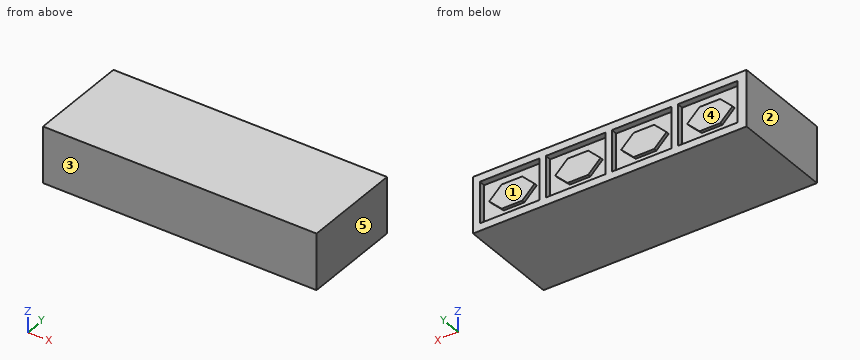
```python
from build123d import *

# Parameters (mm, degrees)
SKETCH2_W           = 132.68
SKETCH2_H           = 48.96
BOSS_EXTRUDE1_DEPTH = 27.2
SKETCH3_W           = 29
SKETCH3_H           = 20
CUT_EXTRUDE1_DEPTH  = 3
SKETCH4_W           = 10
SKETCH4_H           = 11.64
BOSS_EXTRUDE2_DEPTH = 1.5
LPATTERN1_COUNT     = 4
LPATTERN1_PITCH     = 32


with BuildPart() as part:
    # Sketch2 → Boss-Extrude1 (new body)
    with BuildSketch(Plane.XY):
        with Locations((66.34, 24.48)):
            Rectangle(SKETCH2_W, SKETCH2_H)
    extrude(amount=BOSS_EXTRUDE1_DEPTH)

    # Sketch3 → Cut-Extrude1 (cut)
    with BuildSketch(Plane(origin=(0, 48.96, 0), x_dir=(1, 0, 0), z_dir=(0, 1, 0))):
        with Locations((18.855, -13.6)):
            Rectangle(SKETCH3_W, SKETCH3_H)
    cut_extrude1 = extrude(amount=-CUT_EXTRUDE1_DEPTH, mode=Mode.SUBTRACT)

    # Sketch4 → Boss-Extrude2 (add)
    with BuildSketch(Plane(origin=(0, 45.96, 0), x_dir=(1, 0, 0), z_dir=(0, 1, 0))):
        Polygon((13.855, -7.78), (7.855, -13.6), (13.855, -19.42), align=None)
        with Locations((18.855, -13.6)):
            Rectangle(SKETCH4_W, SKETCH4_H)
        Polygon((29.855, -13.6), (23.855, -19.42), (23.855, -7.78), align=None)
    boss_extrude2 = extrude(amount=BOSS_EXTRUDE2_DEPTH)

    # LPattern1: Cut-Extrude1, Boss-Extrude2 ×4
    with Locations(*[(i * LPATTERN1_PITCH, 0, 0) for i in range(1, LPATTERN1_COUNT)]):
        add(cut_extrude1, mode=Mode.SUBTRACT)
        add(boss_extrude2)


solid = part.part
```
Geometry: final body of the model. Coordinates: model frame, mm. Face numbers are marked on the shaded views. A direction names the side the tool comes from. Coordinates: 2 decimals unless noted, no trailing zeros. Write each loop counter-clockwise with the first axis right and the second up, starting at its lowest first coordinate (ties: lowest second). Pieces come first, ordered by that corner, then holes. Notation, with made-up numbers: M 39.25,-33 L 68.25,-33 A16 cw 68.25,-19 Z; hole C -30,-37 d10. An arc over 180 degrees is marked long. Use CSV: the item, a comma, the result in double quotes. Start each with the question number.
1. Mould query, pull axis X, two halves, no side actions, for the marked faces 3, 4 and 5. Classes: pulls with the +X half, pulls with the -X half, needs draft (parallel to the pull), parting line crosses it, or undercut.
2. First-contact query: P1, Ø6, axis at x = 46.5, z = 13.5, coming from the +Y side. Flat tip, straight axial feed; report the tip coordinate or a pass-through.
3. Cut plane A-A on x = 16. Return the cut outline in (y, z).
4. Cut plane C-C on x = 59. Return the cut outline in (y, z).
5. Ray query, probe 1 along X at (y, z) = (46, 7.25) (3 decimals); probe 2 along Y at (x, z) = (122, 23); probe 3 along Y at (x, z) = (85, 19). Return the intervals inside material, ascending.
6. Cut plane B-B on z = 22. Return the cut outline in (x, y) (3 decimals), plus the area to 3 significant figures.
7. Reachability of the marked faces 1 and 2 from +Z, -Z, +X, -X, +Y, -Y: full face, straight path, thin tool, end or side. Return the list, or none.
Entries:
1,face 3,"needs draft"
1,face 4,"undercut"
1,face 5,"pulls with the +X half"
2,P1,"y = 47.46"
3,outline,"M 0,0 L 48.96,0 L 48.96,3.6 L 45.96,3.6 L 45.96,7.78 L 47.46,7.78 L 47.46,19.42 L 45.96,19.42 L 45.96,23.6 L 48.96,23.6 L 48.96,27.2 L 0,27.2 Z"
4,outline,"M 0,0 L 48.96,0 L 48.96,3.6 L 45.96,3.6 L 45.96,10.83 L 47.46,10.83 L 47.46,16.37 L 45.96,16.37 L 45.96,23.6 L 48.96,23.6 L 48.96,27.2 L 0,27.2 Z"
5,probe 1,"0 to 4.355, 33.355 to 36.355, 65.355 to 68.355, 97.355 to 100.355, 129.355 to 132.68"
5,probe 2,"0 to 45.96"
5,probe 3,"0 to 47.46"
6,outline,"M 0,0 L 132.68,0 L 132.68,48.96 L 129.355,48.96 L 129.355,45.96 L 100.355,45.96 L 100.355,48.96 L 97.355,48.96 L 97.355,45.96 L 68.355,45.96 L 68.355,48.96 L 65.355,48.96 L 65.355,45.96 L 36.355,45.96 L 36.355,48.96 L 33.355,48.96 L 33.355,45.96 L 4.355,45.96 L 4.355,48.96 L 0,48.96 Z"
6,area,"6,150 mm²"
7,face 1,"+Y"
7,face 2,"+Z, -Z, -X, +Y, -Y"
